Could you check a few things on this model? Use its own coordinates, in mm. Coordinates: 2 decimals unless noted, no trailing zeros. Write each loop counter-clockwise with the first axis right and the second up, starting at its lowest first coordinate (ties: lowest second). Pieces come first, ordered by that corner, then holes.
Item 1: If I drill on probe 1 along Z at (x, y) = (-62, 26); probe 2 along X at (y, z) = (68, 90); probe 3 along X at (y, z) = (15.5, -1), over which ranges is the centre line in solid material (lowest first)?
Item 2: I want a section at A-A on y = 60.5. Please give me the cut outline in (x, z).
Item 3: I want a section at C-C on z = 60.5. Please give me the cut outline in (x, y).
Item 4: I want a section at B-B on x = -85. Please give me the cut outline in (y, z), then the cut area to 3 significant figures.
Item 5: For P1, Ø3, axis at x = 77, z = 70, coming from the +Y side; P2, Ø1.5, axis at x = 13, z = -47.5, coming from the +Y side, each with a flat end and sliding along its axis, tell me the tip position at first contact or that it passes through.
Item 6: I want a section at D-D on y = 20.5. Please give me the cut outline in (x, z), then the cut area to 3 significant figures.
from build123d import *

# Parameters (mm, degrees)
SKETCH1_W           = 238.3
SKETCH1_H           = 238.3
BOSS_EXTRUDE1_DEPTH = 72.766666667


with BuildPart() as part:
    # Sketch1 → Boss-Extrude1 (new body)
    with BuildSketch(Plane(origin=(0, 0, 0), x_dir=(1, 0, 0), z_dir=(0, 1, 0))):
        Rectangle(SKETCH1_W, SKETCH1_H)
    extrude(amount=BOSS_EXTRUDE1_DEPTH)

    # Sketch3 → Cut-Revolve8 (revolve, cut)
    with BuildSketch(Plane.XY):
        with BuildLine():
            Line((-109.15, 72.766666667), (0, 72.766666667))
            Line((0, 72.766666667), (0, 10))
            Line((0, 10), (0, 0.553473444))
            ThreePointArc((0, 0.553473444), (-65.437886151, 20.240853976), (-109.15, 72.766666667))
        make_face()
    revolve(axis=Axis((0, 72.766666667, 0), (0, -1, 0)), mode=Mode.SUBTRACT)


solid = part.part
Response values:
1. probe 1: z = -119.15 to -39.3, 39.3 to 119.15
1. probe 2: x = -119.15 to -57.87, 57.87 to 119.15
1. probe 3: x = -119.15 to -57.63, 57.63 to 119.15
2. outline: (-119.15, -119.15) - (119.15, -119.15) - (119.15, 119.15) - (-119.15, 119.15) - close; hole circle Ø206.16 at (0, 0)
3. outline: (-119.15, 0) - (119.15, 0) - (119.15, 72.77) - (90.85, 72.77) arc R102 cw to (-90.85, 72.77) - (-119.15, 72.77) - close
4. outline: (0, -119.15) - (72.77, -119.15) - (72.77, -68.47) arc R82.71 cw to (72.77, 68.47) - (72.77, 119.15) - (0, 119.15) - close
4. area: 13,800 mm2
5. P1: stops at y = 65.1
5. P2: stops at y = 11.61
6. outline: (-119.15, -119.15) - (119.15, -119.15) - (119.15, 119.15) - (-119.15, 119.15) - close; hole circle Ø131.66 at (0, 0)
6. area: 43,200 mm2
